Input: dimensioned drawing with shaded views. Units: mm. Origin: part minimum x, y, z. Coordinates: 2 decimals unless noted, no trailing zeros. Loops run counter-clockwise (first coordinate to the right, second up) from the corner with the lowest first, then second, coordinate; pieces in that order, holes last. Notation, with made-up numbers: (81.25, 35.25) - (127.25, 35.25) arc R33 cw to (127.25, 72.25) - close; hole circle Ø10 at (38, 65.25). An arc over 180 degrees is marked (long way). Write item = value, one per line. Start each with the question number.
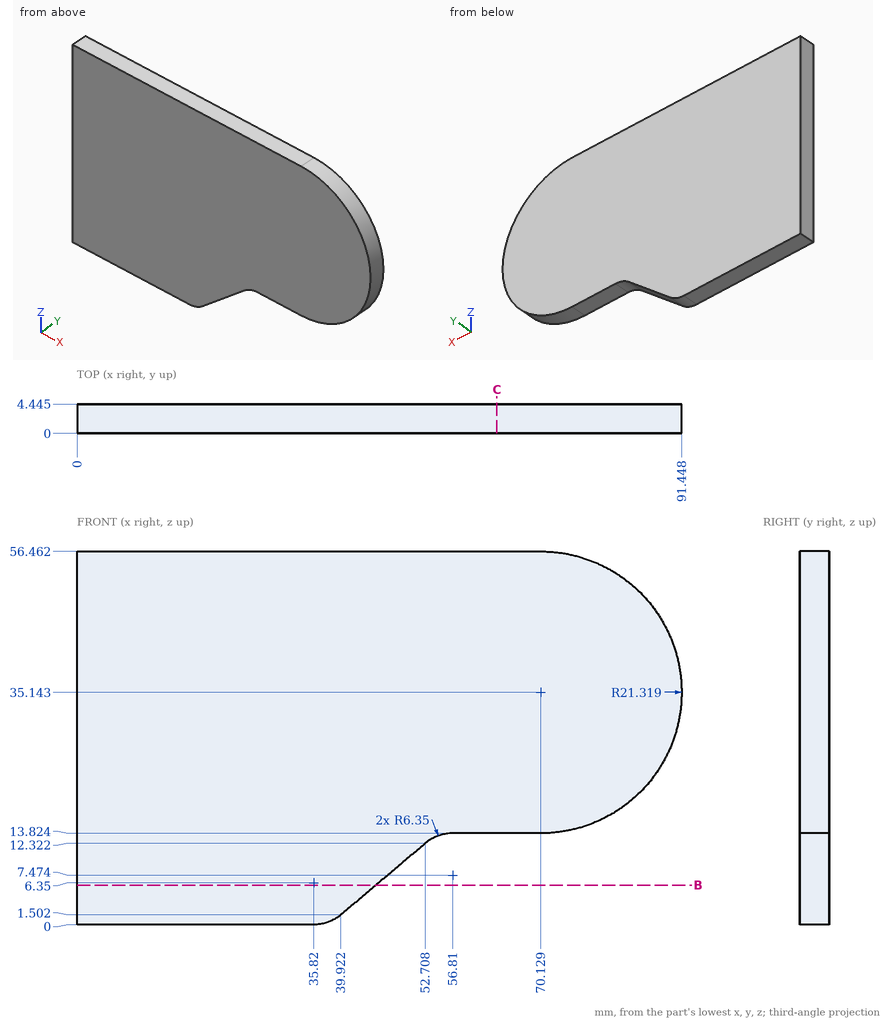
Item 1: Pin query (flat end, axial travel): pin 1 (1.3 mm diameter, centred on x = 64.5, y = 2.5, fed in from -Z); pin 2 (1 mm diameter, centred on x = 71, z = 12.5, fed in from +Y); pin 3 (2 mm diameter, centred on x = 78, y = 3.5, fed in from +Z) (1 decimal). Return the tip coordinate at first contact, or that it passes through.
Item 2: Cut plane C-C on x = 63.5. Return loops of the section in (y, z) (1 decimal).
Item 3: Cut plane B-B on z = 6. Return loops of the section in (x, y) (1 decimal).
Item 4: Ray query, line 1 (Z direction, x = 57, y = 3.9) (1 decimal); line 2 (X direction, y = 2.45, z = 36); line 3 (Z direction, x = 78, y = 3.8) (1 decimal). Return the intervals inside material, ascending.
Recorded:
q1.pin_1 = 13.82
q1.pin_2 = through
q1.pin_3 = 55.3
q2.outline = (0, 13.8) - (4.4, 13.8) - (4.4, 56.5) - (0, 56.5) - close
q3.outline = (0, 0) - (45.2, 0) - (45.2, 4.4) - (0, 4.4) - close
q4.line_1 = 13.8 to 56.5
q4.line_2 = 0 to 91.43
q4.line_3 = 15.3 to 55
